For this review, take the finished solid that the model builds, in its own axes (mm). Face numbers are marked on the shaded views. Round coordinates to 2 decimals unless told otherwise and drop trailing zeros. Write each loop counter-clockwise with the first axis right and the second up, starting at its lowest first coordinate (ties: lowest second). Pieces come first, ordered by that corner, then holes. Notation, with made-up numbers: M -27.75,66.5 L -10.75,66.5 A18 ccw -10.75,83.5 Z; hole C 48,-10.5 d7. An arc over 180 degrees is marked long. Answer in a Markdown table with one row per item.
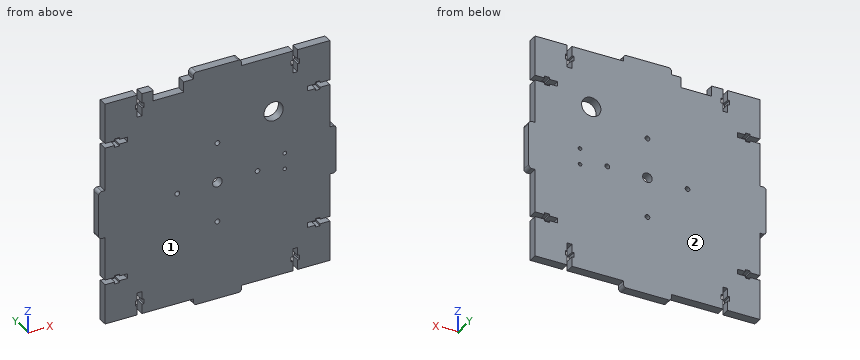
```python
from build123d import *

# Parameters (mm, degrees)
SKETCH1_R           = 3
SKETCH1_R_2         = 1.5
SKETCH1_R_3         = 6
SKETCH1_R_4         = 1.125
BOSS_EXTRUDE1_DEPTH = 5.5
FILLET1_R           = 2


with BuildPart() as part:
    # Sketch1 → Boss-Extrude1 (new body)
    with BuildSketch(Plane(origin=(0, 0, 0), x_dir=(1, 0, 0), z_dir=(0, 1, 0))):
        Polygon((85, 0), (117, 0), (117, 6), (115.8, 6), (115.8, 9), (117, 9), (117, 14), (120, 14), (120, 9), (121.2, 9), (121.2, 6), (120, 6), (120, 0), (140, 0), (140, 25), (134, 25), (134, 23.8), (131, 23.8), (131, 25), (126, 25), (126, 28), (131, 28), (131, 29.2), (134, 29.2), (134, 28), (140, 28), (140, 55), (144, 55), (144, 85), (140, 85), (140, 112), (134, 112), (134, 110.8), (131, 110.8), (131, 112), (126, 112), (126, 115), (131, 115), (131, 116.2), (134, 116.2), (134, 115), (140, 115), (140, 140), (120, 140), (120, 134), (121.2, 134), (121.2, 131), (120, 131), (120, 126), (117, 126), (117, 131), (115.8, 131), (115.8, 134), (117, 134), (117, 140), (85, 140), (85, 144), (55, 144), (55, 140), (23, 140), (23, 134), (24.2, 134), (24.2, 131), (23, 131), (23, 126), (20, 126), (20, 131), (18.8, 131), (18.8, 134), (20, 134), (20, 140), (0, 140), (0, 115), (6, 115), (6, 116.2), (9, 116.2), (9, 115), (14, 115), (14, 112), (9, 112), (9, 110.8), (6, 110.8), (6, 112), (0, 112), (0, 85), (-4, 85), (-4, 55), (0, 55), (0, 28), (6, 28), (6, 29.2), (9, 29.2), (9, 28), (14, 28), (14, 25), (9, 25), (9, 23.8), (6, 23.8), (6, 25), (0, 25), (0, 0), (20, 0), (20, 6), (18.8, 6), (18.8, 9), (20, 9), (20, 14), (23, 14), (23, 9), (24.2, 9), (24.2, 6), (23, 6), (23, 0), (30, 0), (30, 6.5), (49, 6.5), (49, 0), (55, 0), (55, -4), (85, -4), align=None)
        with Locations(Location((70, 70, 0), (0, 0, 270))):
            Circle(SKETCH1_R, mode=Mode.SUBTRACT)
        with Locations(Location((70, 95, 0), (0, 0, 270))):
            Circle(SKETCH1_R_2, mode=Mode.SUBTRACT)
        with Locations(Location((95, 70, 0), (0, 0, 270))):
            Circle(SKETCH1_R_2, mode=Mode.SUBTRACT)
        with Locations(Location((70, 45, 0), (0, 0, 270))):
            Circle(SKETCH1_R_2, mode=Mode.SUBTRACT)
        with Locations(Location((45, 70, 0), (0, 0, 270))):
            Circle(SKETCH1_R_2, mode=Mode.SUBTRACT)
        with Locations(Location((105, 35, 0), (0, 0, 270))):
            Circle(SKETCH1_R_3, mode=Mode.SUBTRACT)
        with Locations(Location((112, 73.556484563, 0), (0, 0, 270))):
            Circle(SKETCH1_R_4, mode=Mode.SUBTRACT)
        with Locations(Location((112, 63.556484563, 0), (0, 0, 270))):
            Circle(SKETCH1_R_4, mode=Mode.SUBTRACT)
    extrude(amount=BOSS_EXTRUDE1_DEPTH)

    # Fillet1
    fillet1_edges = [part.edges().sort_by_distance(p)[0] for p in [
        (-4, 2.75, -55),
        (-4, 2.75, -85),
        (55, 2.75, -144),
        (85, 2.75, -144),
        (144, 2.75, -85),
        (144, 2.75, -55),
        (85, 2.75, 4),
        (55, 2.75, 4),
    ]]
    fillet(fillet1_edges, radius=FILLET1_R)


solid = part.part
```
Q1. Take a section at A-A (x = 105). State the section outline as (y, z) points.
Found:
| item | result |
|---|---|
| outline | M 0,-140 L 5.5,-140 L 5.5,-41 L 0,-41 Z; M 0,-29 L 5.5,-29 L 5.5,0 L 0,0 Z |
Q2. Take a section at B-B (y = 1.6). State how many separate pieces and enclosed holes the cut face has, then the cut area to 3 significant figures.
Found:
| item | result |
|---|---|
| separate pieces | 1 |
| enclosed holes | 8 |
| area | 19,400 mm² |
Q3. Mouldability with a two-part tool opening along Y and no side actions: class the marked faces 1 and 2 as +Y half, -Y half, draft (parallel to the pull), parting line (faces both ways), or undercut.
Found:
| item | result |
|---|---|
| face 1 | -Y half |
| face 2 | +Y half |
Q4. For probe 1 along X at (y, z) = (3.8, -70); probe 2 along Z at (x, y) = (136, 1.2); probe 3 along Z at (x, y) = (24, 4.35), list the stretches that pass through material, from the lowest coordinate up.
Found:
| item | result |
|---|---|
| probe 1 | -4 to 43.5, 46.5 to 67, 73 to 93.5, 96.5 to 144 |
| probe 2 | -140 to -115, -112 to -28, -25 to 0 |
| probe 3 | -140 to -134, -131 to -9, -6 to 0 |
Q5. Take a section at C-C (z = -104.5). State the section outline as (x, y) points, then the cut area to 3 significant figures.
Found:
| item | result |
|---|---|
| outline | M 0,0 L 140,0 L 140,5.5 L 0,5.5 Z |
| area | 770 mm² |
Q6. Insertion check: P1, Ø2.5, axis at y = 1.5, z = -11, coming from the -X side; P2, Ø1.5, axis at x = 44.5, y = 3.5, coming from the -Z side; P3, Ø1.5, axis at x = 18, y = 2.5, coming from the +Z side. Each pin has a flat end and moves straight along its axis. Give the tip position at first contact, or say it passes through.
Found:
| item | result |
|---|---|
| P1 | x = 0 |
| P2 | z = -140 |
| P3 | z = 0 |
Q7. Take a section at D-D (x = 35). State the section outline as (y, z) points, then the cut area to 3 significant figures.
Found:
| item | result |
|---|---|
| outline | M 0,-140 L 5.5,-140 L 5.5,-6.5 L 0,-6.5 Z |
| area | 734 mm² |
